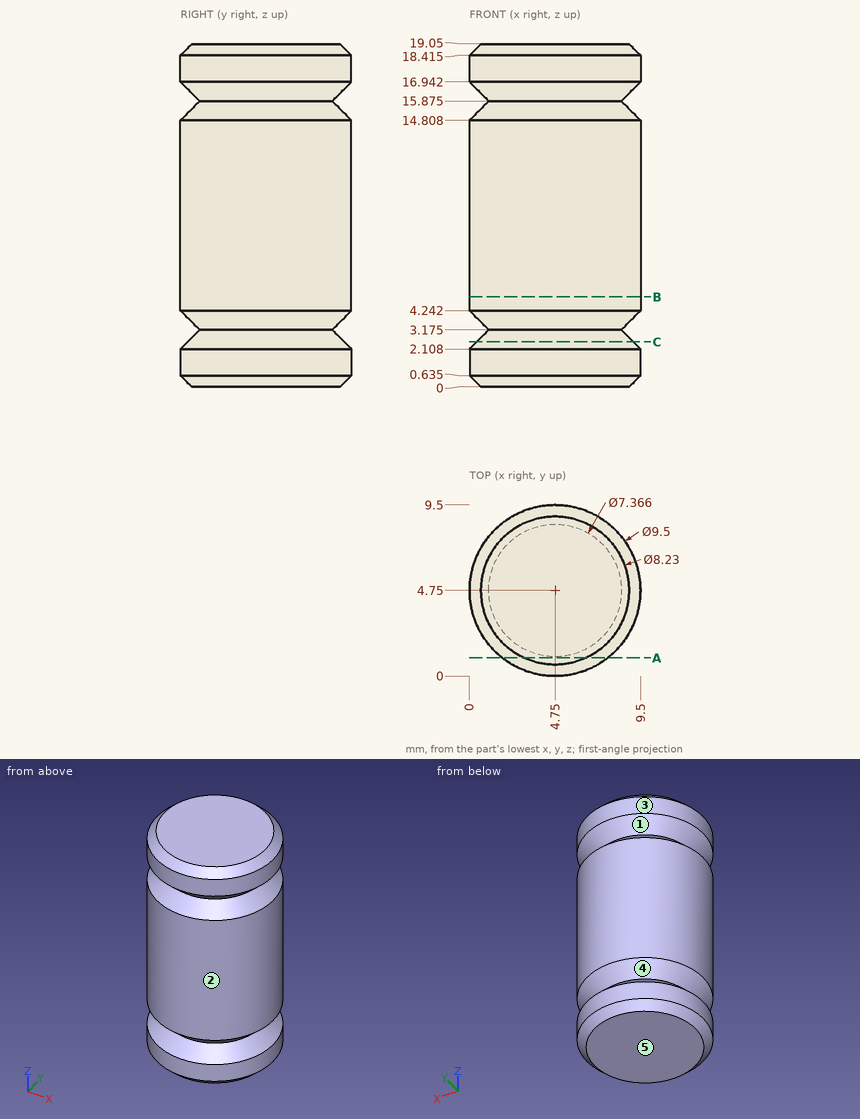
Could you check a few things on this drawing? It's one solid part, dimensions in mm from its lowest x, y, z. A direction names the side the tool comes from. Give positions to 0.01 mm unless a question says otherwise; leave off trailing zeros. Order: outer loops, then holes, each group sorted by start corner. A loop starts at its lowest first (then second) coordinate and runs counter-clockwise, first axis right, second up. Notation, with made-up numbers: M 25,6.5 L 30,6.5 A20 ccw 30,25.5 Z; hole C 1,41 d5. An arc over 180 degrees is marked long. Use one line per item in the form item = value. Start each with the question number.
Item 1: If we section it at A-A (y = 1): State how many separate pieces and enclosed holes the cut face has.
Item 2: We'd pull the mould along Z, two halves only. Please class the marked faces 3, 4 and 5: +Z half, -Z half, draft (parallel to the pull), parting line (faces both ways), or undercut.
Item 3: Will this pin go through, and if not, where does the flat tip stop? pin 1 Ø2 at (y, z) = (8.5, 4) entering from -X.
Item 4: If I drill on line 1 along Z through (x, y) = (6.25, 0.75) (1 decimal); line 2 along Z through (x, y) = (3.25, 1); line 3 along X through (y, z) = (3.5, 13.5), over which ranges is the centre line in solid material (lowest first)?
Item 5: For the marked faces 1 and 2, which set-ups out of +Z, -Z, +X, -X, +Y, -Y let a thin tool reach every point of the face, with its end or its side?
Item 6: If we section it at B-B (z = 5): Write out the boundary of the cut face in (x, y).
Item 7: If we section it at C-C (z = 2.5): Write out the boundary of the cut face in (x, y).
Outcome:
q1.separate_pieces = 3
q1.enclosed_holes = 0
q2.face_3 = draft
q2.face_4 = undercut
q2.face_5 = -Z half
q3.pin_1 = 0.9
q4.line_1 = 0.2 to 2.6, 3.8 to 15.3, 16.5 to 18.9
q4.line_2 = 0 to 2.82, 3.53 to 15.52, 16.23 to 19.05
q4.line_3 = 0.17 to 9.33
q5.face_1 = none
q5.face_2 = +Z, -Z
q6.outline = C 4.75,4.75 d9.5
q7.outline = C 4.75,4.75 d8.72
